Could you check a few things on this model? Use its own coordinates, in mm. A direction names the side the tool comes from. Give positions to 0.01 mm unless a question says otherwise; leave off trailing zeros. Loops run counter-clockwise (first coordinate to the right, second up) from the corner with the lowest first, then second, coordinate; pieces in that order, holes last. Notation, with made-up numbers: (21, 56.5) -> (32, 56.5) arc R25 ccw to (32, 83.5) -> close; hole circle Ø3 at (10.25, 13.5). An arc over 180 degrees is marked (long way). Put each result on its own line as item: value.
```python
from build123d import *

# Parameters (mm, degrees)
SKETCH1_W           = 20
SKETCH1_H           = 18
BOSS_EXTRUDE1_DEPTH = 16.5
CUT_EXTRUDE1_REACH  = 22
SKETCH2_W           = 15
SKETCH2_H           = 15


with BuildPart() as part:
    # Sketch1 → Boss-Extrude1 (new body)
    with BuildSketch(Plane(origin=(0, 0, 0), x_dir=(1, 0, 0), z_dir=(0, 1, 0))):
        Rectangle(SKETCH1_W, SKETCH1_H)
    extrude(amount=BOSS_EXTRUDE1_DEPTH)

    # Sketch2 → Cut-Extrude1 (cut, up to next)
    with BuildSketch(Plane.ZY.offset(10), mode=Mode.PRIVATE) as cut_extrude1_sk1:
        with Locations((0, 7.5)):
            Rectangle(SKETCH2_W, SKETCH2_H)
    cut_extrude1_tool1 = extrude(cut_extrude1_sk1.sketch, amount=-CUT_EXTRUDE1_REACH, mode=Mode.PRIVATE) & part.part
    add(cut_extrude1_tool1.solids().sort_by_distance((-10, 7.5, 0))[0], mode=Mode.SUBTRACT)


solid = part.part
```
1. Thinking about a two-plate mould opening in Z: for faces 3 (the face through (0, 7, 7.5)), 4 (the face through (0, 8, 9)), 5 (the face through (0, 0, -8)), which applies, pulls with the +Z half, pulls with the -Z half, needs draft (parallel to the pull), parting line crosses it, or undercut?
Recorded:
face 3: undercut
face 4: pulls with the +Z half
face 5: needs draft
2. If we section it at B-B (x = 6.5): List the corners of the cut face in (y, z) for me, then the cut area to 3 significant figures.
Recorded:
outline: (0, -9) -> (16.5, -9) -> (16.5, 9) -> (0, 9) -> (0, 7.5) -> (15, 7.5) -> (15, -7.5) -> (0, -7.5) -> close
area: 72.0 mm^2
3. If we section it at A-A (y = 10): List the corners of the cut face in (x, z) for me, then the cut area to 3 significant figures.
Recorded:
outline: (-10, -9) -> (10, -9) -> (10, -7.5) -> (-10, -7.5) -> close; (-10, 7.5) -> (10, 7.5) -> (10, 9) -> (-10, 9) -> close
area: 60.0 mm^2
4. I'm going to push a flat-ended pin straight in: pin 1 (4.5 mm diameter, centred on x = 2.5, z = 2.5, fed in from -Y). Where does the tip first touch, or does it pass through?
Recorded:
pin 1: stops at y = 15
5. For faces 1 (the face through (0, 7, -7.5)), 2 (the face through (-10, 16, 0)), which set-ups out of +Z, -Z, +X, -X, +Y, -Y let a thin tool reach every point of the face, with its end or its side?
Recorded:
face 1: +X, -X, -Y
face 2: +Z, -Z, -X, +Y, -Y
6. I need wall thicknesses on line 1 (Z direction, x = -7, y = 3.25); line 2 (Y direction, x = 8.5, z = -1). Which ranges of each line are inside material? Lowest first, please.
Recorded:
line 1: z = -9 to -7.5, 7.5 to 9
line 2: y = 15 to 16.5
7. If we section it at C-C (z = 5.5): List the corners of the cut face in (x, y) for me, then the cut area to 3 significant figures.
Recorded:
outline: (-10, 15) -> (10, 15) -> (10, 16.5) -> (-10, 16.5) -> close
area: 30.0 mm^2
